```python
from build123d import *

# Parameters (mm, degrees)
BOSS_EXTRUDE1_DEPTH = 1
SKETCH3_W           = 41
SKETCH3_H           = 18
BOSS_EXTRUDE2_DEPTH = 13
SKETCH4_W           = 5.527991342
SKETCH4_H           = 4.817179588
BOSS_EXTRUDE3_DEPTH = 3
SKETCH5_W           = 6
SKETCH5_H           = 2
BOSS_EXTRUDE4_DEPTH = 9
SKETCH6_R           = 4
BOSS_EXTRUDE5_DEPTH = 14
SKETCH7_W           = 2
SKETCH7_H           = 10
BOSS_EXTRUDE6_DEPTH = 14


with BuildPart() as part:
    # Sketch2 → Boss-Extrude1 (new body)
    with BuildSketch(Plane(origin=(0, 0, 0), x_dir=(1, 0, 0), z_dir=(0, 1, 0))):
        Polygon((0, 32), (0, 0), (69, 0), (69, 50), (23, 50), (23, 32), align=None)
    extrude(amount=BOSS_EXTRUDE1_DEPTH)

    # Sketch3 → Boss-Extrude2 (add)
    with BuildSketch(Plane(origin=(0, 1, 0), x_dir=(1, 0, 0), z_dir=(0, 1, 0))):
        with Locations((24.5, 16)):
            Rectangle(SKETCH3_W, SKETCH3_H)
    extrude(amount=BOSS_EXTRUDE2_DEPTH)

    # Sketch4 → Boss-Extrude3 (add)
    with BuildSketch(Plane(origin=(0, 14, 0), x_dir=(1, 0, 0), z_dir=(0, 1, 0))):
        with Locations((6.763995671, 16)):
            Rectangle(SKETCH4_W, SKETCH4_H)
    extrude(amount=BOSS_EXTRUDE3_DEPTH)

    # Sketch5 → Boss-Extrude4 (add)
    with BuildSketch(Plane(origin=(0, 1, 0), x_dir=(1, 0, 0), z_dir=(0, 1, 0))):
        with Locations((42, 3)):
            Rectangle(SKETCH5_W, SKETCH5_H)
    extrude(amount=BOSS_EXTRUDE4_DEPTH)

    # Sketch6 → Boss-Extrude5 (add)
    with BuildSketch(Plane(origin=(0, 1, 0), x_dir=(1, 0, 0), z_dir=(0, 1, 0))):
        with Locations(Location((48, 46, 0), (0, 0, 90))):
            Circle(SKETCH6_R)
    extrude(amount=BOSS_EXTRUDE5_DEPTH)

    # Sketch7 → Boss-Extrude6 (add)
    with BuildSketch(Plane(origin=(0, 1, 0), x_dir=(1, 0, 0), z_dir=(0, 1, 0))):
        with Locations((54.368547089, 43)):
            Rectangle(SKETCH7_W, SKETCH7_H)
    extrude(amount=BOSS_EXTRUDE6_DEPTH)


solid = part.part
```
The listing builds one solid part. Answer for the finished solid, in the listing's coordinates (mm). A direction names the side the tool comes from. Give positions to 0.01 mm unless a question says otherwise; leave off trailing zeros. Order: outer loops, then holes, each group sorted by start corner. A loop starts at its lowest first (then second) coordinate and runs counter-clockwise, first axis right, second up.
1) Consider line 1 along Y through (x, z) = (45.5, -31); line 2 along Z through (x, y) = (10.5, 9.25); line 3 along X through (y, z) = (5.25, -16.5). Determine where each line is inside the solid, lowest interval first.
Reported:
line 1: y = 0 to 1
line 2: z = -25 to -7
line 3: x = 4 to 45
2) Given P1, Ø0.6, axis at x = 41, z = -3, coming from the +Y side; P2, Ø2, axis at x = 54, y = 5.5, coming from the +Z side; P3, Ø2, axis at y = 5.5, z = -2.5, coming from the +X side, each flat-ended and moving along its own axis, determine where each tip first touches the part or whether it passes through.
Reported:
P1: stops at y = 10
P2: stops at z = -38
P3: stops at x = 45
3) Find section D-D on x = 46.5. Write down the section's boundary in (y, z), then the cut area to 3 significant figures.
Reported:
outline: (0, -50) - (1, -50) - (1, -49.71) - (15, -49.71) - (15, -42.29) - (1, -42.29) - (1, 0) - (0, 0) - close
area: 154 mm2
4) Find section A-A on y = 8. Write down the section's boundary in (x, z).
Reported:
outline: (4, -25) - (45, -25) - (45, -7) - (4, -7) - close; (39, -4) - (45, -4) - (45, -2) - (39, -2) - close; circle Ø8 at (48, -46); (53.37, -48) - (55.37, -48) - (55.37, -38) - (53.37, -38) - close
5) Find section B-B on z = -46. Write down the section's boundary in (x, y), then the cut area to 3 significant figures.
Reported:
outline: (23, 0) - (69, 0) - (69, 1) - (55.37, 1) - (55.37, 15) - (53.37, 15) - (53.37, 1) - (52, 1) - (52, 15) - (44, 15) - (44, 1) - (23, 1) - close
area: 186 mm2
6) Find section C-C on x = 19. Write down the section's boundary in (y, z).
Reported:
outline: (0, -32) - (1, -32) - (1, -25) - (14, -25) - (14, -7) - (1, -7) - (1, 0) - (0, 0) - close
7) For faces 1 (the face through (54, 8, -38)), 2 (the face through (42, 5, -4)), 3 (the face through (9.528, 15, -16)), determine the directions among +Z, -Z, +X, -X, +Y, -Y from which every point of the face is accessible in a straight line to the end or side of a thin tool.
Reported:
face 1: +Z, +X, -X, +Y
face 2: +X, -X, +Y
face 3: +Z, -Z, +X, +Y
8) Determine the mould class of faces 4 (the face through (45, 5, -3)), 5 (the face through (53.369, 8, -43)), 6 (the face through (7, 15, -18.409)), 7 (the face through (4, 7, -16)) for opening direction X: pulls with the +X half, pulls with the -X half, needs draft (parallel to the pull), parting line crosses it, or undercut.
Reported:
face 4: pulls with the +X half
face 5: undercut
face 6: needs draft
face 7: pulls with the -X half
